Check sheet for the modelled part. Datum: model origin and axes. Units: mm. Face numbers are marked on the shaded views. Give positions to 0.01 mm unless a question says otherwise; leave off trailing zeros. Order: outer loops, then holes, each group sorted by start corner. A loop starts at its lowest first (then second) coordinate and runs counter-clockwise, first axis right, second up.
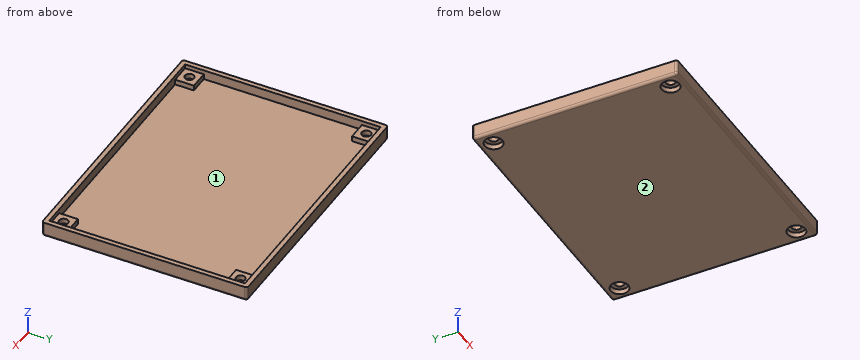
```python
from build123d import *

# Parameters (mm, degrees)
SKETCH_W        = 99.6
SKETCH_H        = 76.6
PAD_DEPTH       = 2
SKETCH001_W     = 99.6
SKETCH001_H     = 76.6
SKETCH001_W_2   = 96
SKETCH001_H_2   = 73
PAD001_DEPTH    = 3.6
SKETCH003_W     = 7
SKETCH003_H     = 7
PAD003_DEPTH    = 2
SKETCH004_R     = 3.3
POCKET_DEPTH    = 2
SKETCH005_R     = 1.7
POCKET001_DEPTH = 5
FILLET_R        = 1
FILLET001_R     = 1
FILLET002_R     = 1
FILLET003_R     = 1
FILLET004_R     = 1


with BuildPart() as part:
    # Sketch → Pad (new body)
    with BuildSketch(Plane.XY):
        with Locations((49.8, 38.3)):
            Rectangle(SKETCH_W, SKETCH_H)
    extrude(amount=PAD_DEPTH)

    # Sketch001 (on Face6 of Pad) → Pad001 (join)
    with BuildSketch(Plane.XY.offset(2)):
        with Locations((49.8, 38.3)):
            Rectangle(SKETCH001_W, SKETCH001_H)
        with Locations((49.8, 38.3)):
            Rectangle(SKETCH001_W_2, SKETCH001_H_2, mode=Mode.SUBTRACT)
    extrude(amount=PAD001_DEPTH)

    # Sketch003 (on Face15 of Pad001) → Pad003 (join)
    with BuildSketch(Plane.XY.offset(2)):
        with Locations((5.3, 5.3)):
            Rectangle(SKETCH003_W, SKETCH003_H)
        with Locations((5.3, 71.3)):
            Rectangle(SKETCH003_W, SKETCH003_H)
        with Locations((94.3, 71.3)):
            Rectangle(SKETCH003_W, SKETCH003_H)
        with Locations((94.3, 5.3)):
            Rectangle(SKETCH003_W, SKETCH003_H)
    extrude(amount=PAD003_DEPTH)

    # Sketch004 (on Face4 of Pad003) → Pocket (cut)
    with BuildSketch(Plane(origin=(0, 0, 0), x_dir=(1, 0, 0), z_dir=(0, 0, -1))):
        with Locations((5.3, -5.3)):
            Circle(SKETCH004_R)
        with Locations((94.3, -5.3)):
            Circle(SKETCH004_R)
        with Locations((5.3, -71.3)):
            Circle(SKETCH004_R)
        with Locations((94.3, -71.3)):
            Circle(SKETCH004_R)
    extrude(amount=-POCKET_DEPTH, mode=Mode.SUBTRACT)

    # Sketch005 (on Face4 of Pocket) → Pocket001 (cut)
    with BuildSketch(Plane(origin=(0, 0, 0), x_dir=(1, 0, 0), z_dir=(0, 0, -1))):
        with Locations((5.3, -5.3)):
            Circle(SKETCH005_R)
        with Locations((5.3, -71.3)):
            Circle(SKETCH005_R)
        with Locations((94.3, -71.3)):
            Circle(SKETCH005_R)
        with Locations((94.3, -5.3)):
            Circle(SKETCH005_R)
    extrude(amount=-POCKET001_DEPTH, mode=Mode.SUBTRACT)

    # Fillet
    fillet_edges = [part.edges().sort_by_distance(p)[0] for p in [
        (0, 76.6, 3.8),
    ]]
    fillet(fillet_edges, radius=FILLET_R)

    # Fillet001
    fillet001_edges = [part.edges().sort_by_distance(p)[0] for p in [
        (0, 0, 2.8),
    ]]
    fillet(fillet001_edges, radius=FILLET001_R)

    # Fillet002
    fillet002_edges = [part.edges().sort_by_distance(p)[0] for p in [
        (99.6, 76.6, 2.8),
    ]]
    fillet(fillet002_edges, radius=FILLET002_R)

    # Fillet003
    fillet003_edges = [part.edges().sort_by_distance(p)[0] for p in [
        (99.6, 0, 2.8),
    ]]
    fillet(fillet003_edges, radius=FILLET003_R)

    # Fillet004
    fillet004_edges = [part.edges().sort_by_distance(p)[0] for p in [
        (49.8, 0, 0),
    ]]
    fillet(fillet004_edges, radius=FILLET004_R)


solid = part.part
```
(1) Release check for a two-part mould opening along X. For the marked faces 1 and 2 record: released by +X, released by -X, zero draft, split by the parting line, or undercut.
(2) Sectioned sample at C-C (y = 50.5). Enter the section's corners in (x, z).
(3) Sectioned sample at A-A (x = 94.3). Count the separate pieces of the cut face and the enclosed holes in it, plus the area to 3 significant figures.
(4) Go/stop test with flat-tipped pins: P1, Ø7.5, axis at x = 94.3, y = 5.3, coming from the -Z side; P2, Ø2, axis at x = 67, y = 49.5, coming from the +Z side. Record where each tip stops, or that it passes through.
(5) Thickness scan on L1, parallel to Y at x = 94.3, z = 3.2; L2, parallel to Y at x = 94.3, z = 1.55; L3, parallel to X at y = 5.3, z = 3. Record the ranges inside material, lowest first.
Values follow:
1. face 1: undercut
1. face 2: zero draft
2. outline: (0, 1) arc R1 ccw to (1, 0) - (98.6, 0) arc R1 ccw to (99.6, 1) - (99.6, 5.6) - (97.8, 5.6) - (97.8, 2) - (1.8, 2) - (1.8, 5.6) - (0, 5.6) - close
3. separate pieces: 3
3. enclosed holes: 0
3. area: 154 mm2
4. P1: stops at z = 0
4. P2: stops at z = 2
5. L1: y = 0 to 3.6, 7 to 8.8, 67.8 to 69.6, 73 to 76.6
5. L2: y = 0 to 2, 8.6 to 68, 74.6 to 76.6
5. L3: x = 0 to 3.6, 7 to 8.8, 90.8 to 92.6, 96 to 99.6
